Work out the finished part from the listing and answer in its coordinate system (mm). A direction names the side the tool comes from. Coordinates: 2 decimals unless noted, no trailing zeros. Loops run counter-clockwise (first coordinate to the right, second up) from the corner with the lowest first, then second, coordinate; pieces in that order, holes last. Notation, with made-up numbers: (-35, 16) -> (-1, 16) arc R20 cw to (-1, 27) -> close; hole circle Ø4 at (66.25, 41). An arc over 180 degrees is marked (long way). Use a Markdown table: item, result.
from build123d import *

# Parameters (mm, degrees)
SKETCH1_W           = 42.5
SKETCH1_H           = 40
BOSS_EXTRUDE1_DEPTH = 2.25
SKETCH3_R           = 6
CUT_EXTRUDE2_DEPTH  = 5
SKETCH4_W           = 42.5
SKETCH4_H           = 4.5
BOSS_EXTRUDE2_DEPTH = 15
SKETCH7_R           = 1.5
CUT_EXTRUDE3_DEPTH  = 10
SKETCH8_W           = 2.5
SKETCH8_H           = 55
CUT_EXTRUDE4_DEPTH  = 10
SKETCH9_W           = 40
SKETCH9_H           = 4.5
BOSS_EXTRUDE3_DEPTH = 110
SKETCH11_R          = 11
CUT_EXTRUDE5_DEPTH  = 100
CUT_EXTRUDE6_DEPTH  = 100


with BuildPart() as part:
    # Sketch1 → Boss-Extrude1 (new, symmetric)
    with BuildSketch(Plane.XY):
        Rectangle(SKETCH1_W, SKETCH1_H)
    extrude(amount=BOSS_EXTRUDE1_DEPTH, both=True)

    # Sketch3 → Cut-Extrude2 (cut, symmetric)
    with BuildSketch(Plane.XY.offset(2.25)):
        with Locations((1.25, 0)):
            Circle(SKETCH3_R)
    extrude(amount=CUT_EXTRUDE2_DEPTH, both=True, mode=Mode.SUBTRACT)

    # Sketch4 → Boss-Extrude2 (add)
    with BuildSketch(Plane(origin=(0, 20, 0), x_dir=(1, 0, 0), z_dir=(0, 1, 0))):
        Rectangle(SKETCH4_W, SKETCH4_H)
    extrude(amount=BOSS_EXTRUDE2_DEPTH)

    # Sketch7 → Cut-Extrude3 (cut)
    with BuildSketch(Plane.XY.offset(2.25)):
        with Locations((-7.75, 24.053632735)):
            Circle(SKETCH7_R)
        with Locations((10.25, 24.053632735)):
            Circle(SKETCH7_R)
        with Locations((10.25, -8.945771811)):
            Circle(SKETCH7_R)
        with Locations((-7.75, -9.053903396)):
            Circle(SKETCH7_R)
    extrude(amount=-CUT_EXTRUDE3_DEPTH, mode=Mode.SUBTRACT)

    # Sketch8 → Cut-Extrude4 (cut)
    with BuildSketch(Plane.XY.offset(2.25)):
        with Locations((-20, 7.5)):
            Rectangle(SKETCH8_W, SKETCH8_H)
    extrude(amount=-CUT_EXTRUDE4_DEPTH, mode=Mode.SUBTRACT)

    # Sketch9 → Boss-Extrude3 (add)
    with BuildSketch(Plane(origin=(0, 35, 0), x_dir=(1, 0, 0), z_dir=(0, 1, 0))):
        with Locations((1.25, 0)):
            Rectangle(SKETCH9_W, SKETCH9_H)
    extrude(amount=BOSS_EXTRUDE3_DEPTH)

    # Sketch11 → Cut-Extrude5 (cut)
    with BuildSketch(Plane(origin=(0, 0, -2.25), x_dir=(-1, 0, 0), z_dir=(0, 0, -1))):
        with Locations((0, 123)):
            Circle(SKETCH11_R)
    extrude(amount=-CUT_EXTRUDE5_DEPTH, mode=Mode.SUBTRACT)

    # Sketch12 → Cut-Extrude6 (cut)
    with BuildSketch(Plane(origin=(0, 0, -2.25), x_dir=(-1, 0, 0), z_dir=(0, 0, -1))):
        with BuildLine():
            Line((18.75, 78.5), (18.75, 86.5))
            Line((18.75, 86.5), (12.247409999, 83.644510066))
            ThreePointArc((12.247409999, 83.644510066), (11.5, 82.499999945), (12.2474101, 81.35548989))
            Line((12.2474101, 81.35548989), (18.75, 78.5))
        make_face()
    extrude(amount=-CUT_EXTRUDE6_DEPTH, mode=Mode.SUBTRACT)


solid = part.part
Q1. Determine the mould class of faces 1 (the flat face through (1, -20, 0)), 2 (the flat face through (-15.54, 85.09, -0.03)), 3 (the flat face through (-18.75, 115, 0)) for opening direction Y: pulls with the +Y half, pulls with the -Y half, needs draft (parallel to the pull), parting line crosses it, or undercut.
Solved:
| item | result |
|---|---|
| face 1 | pulls with the -Y half |
| face 2 | undercut |
| face 3 | needs draft |
Q2. Section A-A on y = 123 is taken. Determine the outline of the cut face in (x, z), and give its area (3 significant figures).
Solved:
| item | result |
|---|---|
| outline | (-18.75, -2.25) -> (-11, -2.25) -> (-11, 2.25) -> (-18.75, 2.25) -> close; (11, -2.25) -> (21.25, -2.25) -> (21.25, 2.25) -> (11, 2.25) -> close |
| area | 81.0 mm² |
Q3. Given pin 1 Ø2.5 at (x, y) = (-7.75, 24.05) entering from +Z; pin 2 Ø3.5 at (x, y) = (10.25, -8.95) entering from +Z, each flat-ended and moving along its own axis, determine where each tip first touches the part or whether it passes through.
Solved:
| item | result |
|---|---|
| pin 1 | through |
| pin 2 | z = 2.25 |
Q4. For faces 4 (the cylindrical face through (-3.51, -3.65, 0.03)), 5 (the flat face through (-15.45, 79.95, -0.03)), determine the directions among +Z, -Z, +X, -X, +Y, -Y from which every point of the face is accessible in a straight line to the end or side of a thin tool.
Solved:
| item | result |
|---|---|
| face 4 | +Z, -Z |
| face 5 | +Z, -Z, -X |
Q5. Section B-B on z = 1.55 is taken. Determine the outline of the cut face in (x, y), and give its area (3 significant figures).
Solved:
| item | result |
|---|---|
| outline | (-18.75, -20) -> (21.25, -20) -> (21.25, 145) -> (-18.75, 145) -> (-18.75, 86.5) -> (-12.25, 83.64) arc R1.25 cw to (-12.25, 81.36) -> (-18.75, 78.5) -> close; hole circle Ø22 at (0, 123); hole circle Ø3 at (-7.75, -9.05); hole circle Ø3 at (-7.75, 24.05); hole circle Ø12 at (1.25, 0); hole circle Ø3 at (10.25, -8.95); hole circle Ø3 at (10.25, 24.05) |
| area | 6,040 mm² |
Q6. Consider line 1 (Y direction, x = 0, z = -0.4); line 2 (Y direction, x = 10, z = 1.9); line 3 (Y direction, x = 1.5, z = 0.45). Determine where each line is inside the solid, lowest interval first. Write a range as [from, to].
Solved:
| item | result |
|---|---|
| line 1 | [-20, -5.87], [5.87, 112], [134, 145] |
| line 2 | [-20, -10.42], [-7.47, 22.57], [25.53, 118.42], [127.58, 145] |
| line 3 | [-20, -5.99], [5.99, 112.1], [133.9, 145] |
Q7. Section C-C on x = 3 is taken. Determine the outline of the cut face in (y, z), and give its area (3 significant figures).
Solved:
| item | result |
|---|---|
| outline | (-20, -2.25) -> (-5.74, -2.25) -> (-5.74, 2.25) -> (-20, 2.25) -> close; (5.74, -2.25) -> (112.42, -2.25) -> (112.42, 2.25) -> (5.74, 2.25) -> close; (133.58, -2.25) -> (145, -2.25) -> (145, 2.25) -> (133.58, 2.25) -> close |
| area | 596 mm² |
Q8. Section D-D on y = 0 is taken. Determine the outline of the cut face in (x, z), and give its area (3 significant figures).
Solved:
| item | result |
|---|---|
| outline | (-18.75, -2.25) -> (-4.75, -2.25) -> (-4.75, 2.25) -> (-18.75, 2.25) -> close; (7.25, -2.25) -> (21.25, -2.25) -> (21.25, 2.25) -> (7.25, 2.25) -> close |
| area | 126 mm² |
